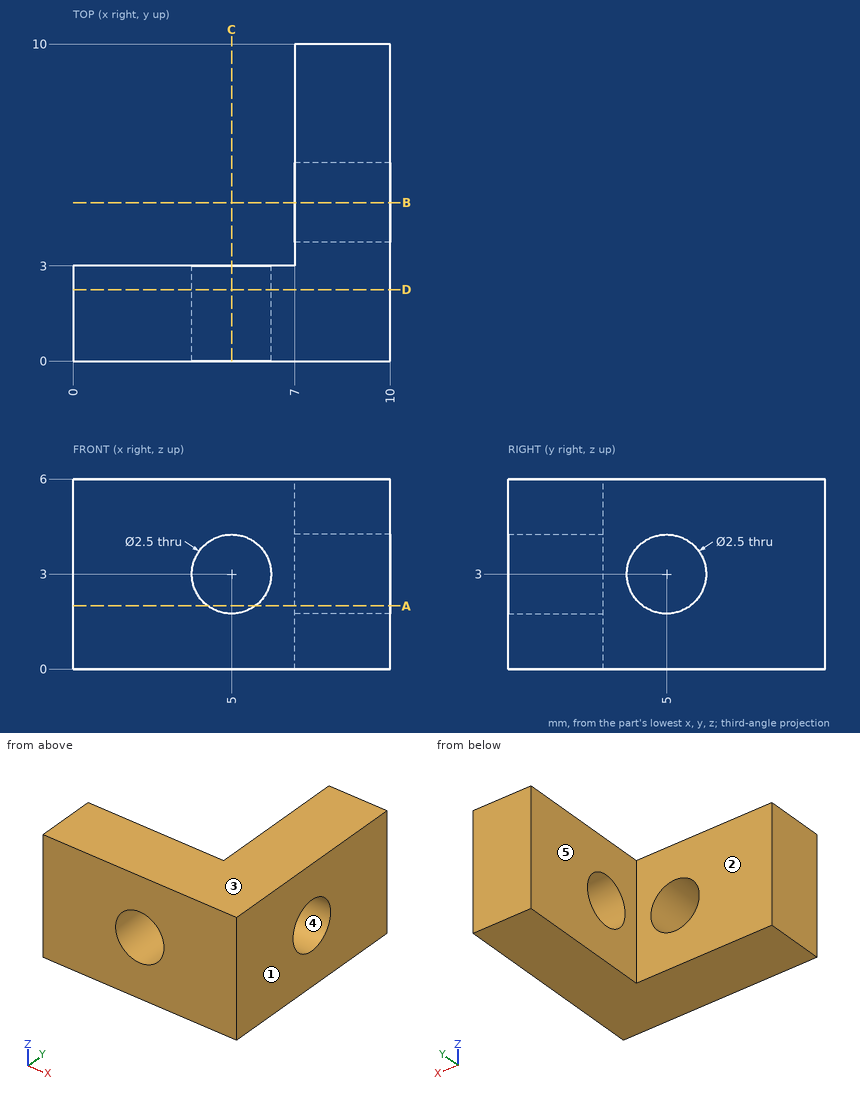
Study the drawing (mm; zero at the part's minimum x, y, z) and answer. A direction names the side the tool comes from. Give positions to 0.01 mm unless a question says otherwise; leave off trailing zeros. Loops run counter-clockwise (first coordinate to the right, second up) from the corner with the lowest first, then second, coordinate; pieces in that order, holes last. Notation, with made-up numbers: (18, 37) - (67, 37) arc R21 cw to (67, 73) - close; hole circle Ø3 at (51.25, -31). An arc over 180 degrees is marked (long way). Return JSON: item names as keys, results as strings. Group by question number.
1. Straight lines are drawn through the part: line 1 (Z direction, x = 5, y = 0.95); line 2 (X direction, y = 3.25, z = 4); line 3 (Y direction, x = 6.75, z = 5.85). For each, find the intervals that lie inside material, in ascending order. Write a range as [from, to].
2. Find section A-A (z = 2). Write down the section's boundary in (x, y).
3. Determine the mould class of the marked faces 3, 4 and 5 for opening direction Z: pulls with the +Z half, pulls with the -Z half, needs draft (parallel to the pull), parting line crosses it, or undercut.
4. Find section D-D (y = 2.25). Write down the section's boundary in (x, z), then the cut area to 3 significant figures.
5. Find section C-C (x = 5). Write down the section's boundary in (y, z), then the cut area to 3 significant figures.
6. Given pin 1 Ø1.5 at (x, z) = (6, 3) entering from +Y, flat-ended and moving along its own axis, determine where the tip first touches the part or whether it passes through.
7. Which of the six approach directions +Z, -Z, +X, -X, +Y, -Y give full straight-line access (tool end or side, diameter ignored) to the marked faces 1 and 2?
8. Find section B-B (y = 5). Write down the section's boundary in (x, z), then the cut area to 3 significant figures.
Verdict:
{
 "1": {"line 1": "z = [0, 1.75], [4.25, 6]", "line 2": "x = [7, 10]", "line 3": "y = [0, 3]"},
 "2": {"outline": "(0, 0) - (4.25, 0) - (4.25, 3) - (0, 3) - close; (5.75, 0) - (10, 0) - (10, 4.25) - (7, 4.25) - (7, 3) - (5.75, 3) - close; (7, 5.75) - (10, 5.75) - (10, 10) - (7, 10) - close"},
 "3": {"face 3": "pulls with the +Z half", "face 4": "undercut", "face 5": "needs draft"},
 "4": {"outline": "(0, 0) - (10, 0) - (10, 6) - (0, 6) - close; hole circle Ø2.5 at (5, 3)", "area": "55.1 mm^2"},
 "5": {"outline": "(0, 0) - (3, 0) - (3, 1.75) - (0, 1.75) - close; (0, 4.25) - (3, 4.25) - (3, 6) - (0, 6) - close", "area": "10.5 mm^2"},
 "6": {"pin 1": "stops at y = 3"},
 "7": {"face 1": "+Z, -Z, +X, +Y, -Y", "face 2": "+Z, -Z, -X, +Y"},
 "8": {"outline": "(7, 0) - (10, 0) - (10, 1.75) - (7, 1.75) - close; (7, 4.25) - (10, 4.25) - (10, 6) - (7, 6) - close", "area": "10.5 mm^2"}
}
